from build123d import *

# Parameters (mm, degrees)
BOSS_EXTRUDE1_DEPTH = 8
SKETCH2_R           = 1.95
CUT_EXTRUDE1_DEPTH  = 150
CUT_EXTRUDE2_DEPTH  = 150
CUT_EXTRUDE3_DEPTH  = 150
FILLET2_R           = 0.5
FILLET3_R           = 2


with BuildPart() as part:
    # Sketch1 → Boss-Extrude1 (new body)
    with BuildSketch(Plane.XY):
        Polygon((50, 45), (-50, 45), (-50, -45), (50, -45), (50, -25), (90, -25), (90, 25), (50, 25), align=None)
    extrude(amount=BOSS_EXTRUDE1_DEPTH)

    # Sketch2 → Cut-Extrude1 (cut)
    with BuildSketch(Plane(origin=(0, 25, 0), x_dir=(1, 0, 0), z_dir=(0, 1, 0))):
        with Locations(Location((84, -4, 0), (0, 0, 180))):
            Circle(SKETCH2_R)
    extrude(amount=-CUT_EXTRUDE1_DEPTH, mode=Mode.SUBTRACT)

    # Sketch3 → Cut-Extrude2 (cut)
    with BuildSketch(Plane(origin=(0, 25, 0), x_dir=(1, 0, 0), z_dir=(0, 1, 0))):
        with BuildLine():
            Line((90, -8), (84, -8))
            ThreePointArc((84, -8), (88, -4), (84, 0))
            Line((84, 0), (90, 0))
            Line((90, 0), (90, -8))
        make_face()
    extrude(amount=-CUT_EXTRUDE2_DEPTH, mode=Mode.SUBTRACT)

    # Sketch4 → Cut-Extrude3 (cut)
    with BuildSketch(Plane(origin=(0, 45, 0), x_dir=(1, 0, 0), z_dir=(0, 1, 0))):
        Polygon((-50, -4), (-40.018576331, 0), (-37.957023518, -4), (-36.018576331, 0), (-33.957023518, -4), (-32.018576331, 0), (-29.957023518, -4), (-28.018576331, 0), (-25.957023518, -4), (-24.018576331, 0), (-21.957023518, -4), (-20.018576331, 0), (-17.957023518, -4), (-16.018576331, 0), (-13.957023518, -4), (-12.018576331, 0), (-9.957023518, -4), (-8.018576331, 0), (-5.957023518, -4), (-4.018576331, 0), (-1.957023518, -4), (-0.018576331, 0), (2.042976482, -4), (3.981423669, 0), (6.042976482, -4), (7.981423669, 0), (10.042976482, -4), (11.981423669, 0), (14.042976482, -4), (15.981423669, 0), (18.042976482, -4), (19.981423669, 0), (22.042976482, -4), (23.981423669, 0), (26.042976482, -4), (27.981423669, 0), (30.042976482, -4), (31.981423669, 0), (34.042976482, -4), (35.981423669, 0), (38.042976482, -4), (39.981423669, 0), (37.159266961, 4.620546543), (-31.267866038, 8.187837837), (-50, 0), align=None)
    extrude(amount=-CUT_EXTRUDE3_DEPTH, mode=Mode.SUBTRACT)

    # Fillet2
    fillet2_edges = [part.edges().sort_by_distance(p)[0] for p in [
        (-40.018576331, 0, 0),
    ]]
    fillet(fillet2_edges, radius=FILLET2_R)

    # Fillet3
    fillet3_edges = [part.edges().sort_by_distance(p)[0] for p in [
        (-50, 0, 4),
    ]]
    fillet(fillet3_edges, radius=FILLET3_R)


solid = part.part
Input: part model. Units: mm. Frame: model coordinates. A direction names the side the tool comes from. Give positions to 0.01 mm unless a question says otherwise; leave off trailing zeros. Write each loop counter-clockwise with the first axis right and the second up, starting at its lowest first coordinate (ties: lowest second). Pieces come first, ordered by that corner, then holes. Notation, with made-up numbers: (34, 17.25) -> (75, 17.25) arc R12 cw to (75, 24.25) -> close; hole circle Ø11 at (88, -16.5). An arc over 180 degrees is marked (long way). Use one line per item in the form item = value. Start each with the question number.
1) Set-up query: faces 4 (the flat face through (50, 35, 4)), 5 (the flat face through (-44.65, 0.63, 1.856)). Return all of +Z, -Z, +X, -X, +Y, -Y with unobstructed straight access to the full face (end or side cutting, diameter ignored); none if empty.
2) Ray query, probe 1 along Z at (x, y) = (84, 13); probe 2 along Y at (x, z) = (72, 4.75); probe 3 along X at (y, z) = (-21, 4.5). Return the intervals inside material, ascending. Write a range as from..to.
3) Pin query (flat end, axial travel): pin 1 (4 mm diameter, centred on y = -32, z = 2.5, fed in from +X); pin 2 (1.5 mm diameter, centred on y = 2, z = 2, fed in from +X); pin 3 (1 mm diameter, centred on x = -23, y = -6, fed in from -Z). Return the tip coordinate at first contact, or that it passes through.
4) Section query A-A on x = 51.5. Return the cut outline in (y, z), then the cut area to 3 significant figures.
5) Draft query along X for faces 1 (the flat face through (26.999, 0.63, 2.028)), 2 (the flat face through (-50, 1, 7)), 3 (the flat face through (69, -25, 4)). Return one class per face: pulls with the +X half, pulls with the -X half, needs draft (parallel to the pull), parting line crosses it, or undercut.
Outcome:
q1.face_4 = +Z, -Z, +X, +Y
q1.face_5 = -Z, -X, +Y, -Y
q2.probe_1 = 0..2.05, 5.95..8
q2.probe_2 = -25..25
q2.probe_3 = -49.81..82.12, 85.88..87.97
q3.pin_1 = 50
q3.pin_2 = 87.8
q3.pin_3 = 1.01
q4.outline = (-25, 0) -> (25, 0) -> (25, 8) -> (-25, 8) -> close
q4.area = 400 mm^2
q5.face_1 = undercut
q5.face_2 = pulls with the -X half
q5.face_3 = needs draft
